Geometry check sheet. Reference: drawing and pictorial views, mm from the part's lowest x, y, z. A direction names the side the tool comes from. Coordinates: 2 decimals unless noted, no trailing zeros. Order: outer loops, then holes, each group sorted by start corner. A loop starts at its lowest first (then second) coordinate and runs counter-clockwise, first axis right, second up. Notation, with made-up numbers: (-11, -10) -> (33, -10) arc R12 ccw to (33, 10) -> close; hole circle Ø4 at (-18, -15). An arc over 180 degrees is marked (long way). Use CSV: the item, a comma, the result in double quotes. Start each with the question number.
1) Go/stop test with flat-tipped pins: pin 1 (0.8 mm diameter, centred on x = 3.5, z = 0.5, fed in from +Y); pin 2 (3 mm diameter, centred on x = 1, z = 0.5, fed in from -Y); pin 3 (3 mm diameter, centred on x = 3, z = 3, fed in from -Y); pin 4 (1.6 mm diameter, centred on x = 2.5, y = 13.5, fed in from -Z). Record where each tip stops, or that it passes through.
2) Sectioned sample at A-A on x = 3. Record the boundary of the cut face in (y, z).
3) Scan lines: line 1 along Y through (x, z) = (0.9, 1.4); line 2 along Y through (x, z) = (0.85, 4.05); line 3 along X through (y, z) = (18.25, 4.2). Record each from-to range of solid material in increasing order.
4) Sectioned sample at C-C on y = 10. Record the boundary of the cut face in (x, z).
5) Sectioned sample at B-B on z = 3. Record the boundary of the cut face in (x, y).
6) Tool access check on the marked faces 1, 2 and 3. Record the directions out of +Z, -Z, +X, -X, +Y, -Y that give a thin tool (end or side, any length) a straight path to the whole face; none if there is none.
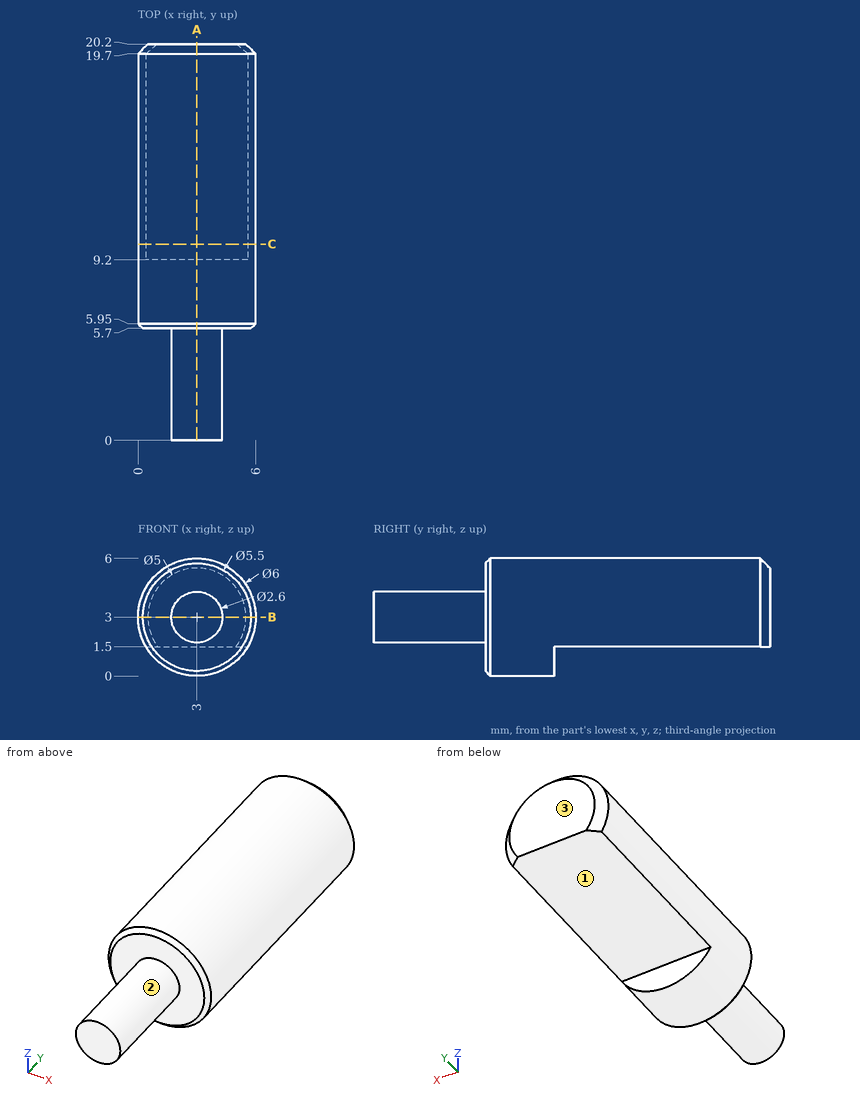
Answers follow:
1,pin 1,"stops at y = 9.2"
1,pin 2,"stops at y = 5.7"
1,pin 3,"stops at y = 0"
1,pin 4,"stops at z = 1.5"
2,outline,"(0, 1.7) -> (5.7, 1.7) -> (5.7, 0.25) -> (5.95, 0) -> (9.2, 0) -> (9.2, 1.5) -> (20.2, 1.5) -> (20.2, 5.5) -> (19.7, 6) -> (5.95, 6) -> (5.7, 5.75) -> (5.7, 4.3) -> (0, 4.3) -> close"
3,line 1,"y = 5.7 to 9.2"
3,line 2,"y = 5.7 to 20.2"
3,line 3,"x = 0.25 to 5.75"
4,outline,"(0.4, 1.5) -> (5.6, 1.5) arc R3 ccw (long way) to start"
5,outline,"(0, 5.95) -> (0.25, 5.7) -> (1.7, 5.7) -> (1.7, 0) -> (4.3, 0) -> (4.3, 5.7) -> (5.75, 5.7) -> (6, 5.95) -> (6, 19.7) -> (5.5, 20.2) -> (0.5, 20.2) -> (0, 19.7) -> close"
6,face 1,"-Z, +X, -X, +Y"
6,face 2,"-Y"
6,face 3,"+Z, -Z, +X, -X, +Y"
